from build123d import *

# Parameters (mm, degrees)
SKETCH1_R           = 3.5
BOSS_EXTRUDE1_DEPTH = 17.78
SKETCH2_R           = 12.192
CUT_EXTRUDE1_DEPTH  = 15.24
CUT_EXTRUDE3_REACH  = 49.719
SKETCH4_W           = 2
SKETCH4_H           = 2
CUT_EXTRUDE4_REACH  = 45.308
SKETCH5_R           = 1.5
SKETCH5_W           = 10
SKETCH5_H           = 25.4
CUT_EXTRUDE5_REACH  = 38.451
SKETCH2_2_R         = 12.192
SKETCH6_R           = 12.192
BOSS_EXTRUDE2_DEPTH = 8
CUT_EXTRUDE6_REACH  = 55.634
SKETCH7_W           = 3
SKETCH7_H           = 3


with BuildPart() as part:
    # Sketch1 → Boss-Extrude1 (new, symmetric)
    with BuildSketch(Plane.XY):
        Polygon((26.938, -11.938), (16.938, -11.938), (16.938, 16.938), (-16.938, 16.938), (-16.938, -11.938), (-26.938, -11.938), (-26.938, -16.938), (26.938, -16.938), align=None)
        Circle(SKETCH1_R, mode=Mode.SUBTRACT)
    extrude(amount=BOSS_EXTRUDE1_DEPTH, both=True)

    # Sketch2 → Cut-Extrude1 (cut, symmetric)
    with BuildSketch(Plane.XY):
        Circle(SKETCH2_R)
    extrude(amount=CUT_EXTRUDE1_DEPTH, both=True, mode=Mode.SUBTRACT)

    # Sketch4 → Cut-Extrude3 (cut, up to next)
    with BuildSketch(Plane.XY.offset(17.78), mode=Mode.PRIVATE) as cut_extrude3_sk1:
        with Locations((-10.219, -1)):
            Rectangle(SKETCH4_W, SKETCH4_H)
    cut_extrude3_tool1 = extrude(cut_extrude3_sk1.sketch, amount=-CUT_EXTRUDE3_REACH, mode=Mode.PRIVATE) & part.part
    # Sketch4 → Cut-Extrude3 (cut, up to next)
    with BuildSketch(Plane.XY.offset(17.78), mode=Mode.PRIVATE) as cut_extrude3_sk2:
        with Locations((10.219, -1)):
            Rectangle(SKETCH4_W, SKETCH4_H)
    cut_extrude3_tool2 = extrude(cut_extrude3_sk2.sketch, amount=-CUT_EXTRUDE3_REACH, mode=Mode.PRIVATE) & part.part
    add(cut_extrude3_tool1.solids().sort_by_distance((-10.219, -1, 17.78))[0], mode=Mode.SUBTRACT)
    add(cut_extrude3_tool2.solids().sort_by_distance((10.219, -1, 17.78))[0], mode=Mode.SUBTRACT)

    # Sketch5 → Cut-Extrude4 (cut, up to next)
    with BuildSketch(Plane(origin=(0, -11.938, 0), x_dir=(1, 0, 0), z_dir=(0, 1, 0)), mode=Mode.PRIVATE) as cut_extrude4_sk1:
        with Locations(Location((-21.938, 15.24, 0), (0, 0, 270))):
            Circle(SKETCH5_R)
    cut_extrude4_tool1 = extrude(cut_extrude4_sk1.sketch, amount=-CUT_EXTRUDE4_REACH, mode=Mode.PRIVATE) & part.part
    # Sketch5 → Cut-Extrude4 (cut, up to next)
    with BuildSketch(Plane(origin=(0, -11.938, 0), x_dir=(1, 0, 0), z_dir=(0, 1, 0)), mode=Mode.PRIVATE) as cut_extrude4_sk2:
        with Locations(Location((21.938, 15.24, 0), (0, 0, 90))):
            Circle(SKETCH5_R)
    cut_extrude4_tool2 = extrude(cut_extrude4_sk2.sketch, amount=-CUT_EXTRUDE4_REACH, mode=Mode.PRIVATE) & part.part
    # Sketch5 → Cut-Extrude4 (cut, up to next)
    with BuildSketch(Plane(origin=(0, -11.938, 0), x_dir=(1, 0, 0), z_dir=(0, 1, 0)), mode=Mode.PRIVATE) as cut_extrude4_sk3:
        with Locations(Location((21.938, -15.24, 0), (0, 0, 270))):
            Circle(SKETCH5_R)
    cut_extrude4_tool3 = extrude(cut_extrude4_sk3.sketch, amount=-CUT_EXTRUDE4_REACH, mode=Mode.PRIVATE) & part.part
    # Sketch5 → Cut-Extrude4 (cut, up to next)
    with BuildSketch(Plane(origin=(0, -11.938, 0), x_dir=(1, 0, 0), z_dir=(0, 1, 0)), mode=Mode.PRIVATE) as cut_extrude4_sk4:
        with Locations(Location((-21.938, -15.24, 0), (0, 0, 90))):
            Circle(SKETCH5_R)
    cut_extrude4_tool4 = extrude(cut_extrude4_sk4.sketch, amount=-CUT_EXTRUDE4_REACH, mode=Mode.PRIVATE) & part.part
    # Sketch5 → Cut-Extrude4 (cut, up to next)
    with BuildSketch(Plane(origin=(0, -11.938, 0), x_dir=(1, 0, 0), z_dir=(0, 1, 0)), mode=Mode.PRIVATE) as cut_extrude4_sk5:
        with Locations((-21.938, 0)):
            Rectangle(SKETCH5_W, SKETCH5_H)
    cut_extrude4_tool5 = extrude(cut_extrude4_sk5.sketch, amount=-CUT_EXTRUDE4_REACH, mode=Mode.PRIVATE) & part.part
    # Sketch5 → Cut-Extrude4 (cut, up to next)
    with BuildSketch(Plane(origin=(0, -11.938, 0), x_dir=(1, 0, 0), z_dir=(0, 1, 0)), mode=Mode.PRIVATE) as cut_extrude4_sk6:
        with Locations((21.938, 0)):
            Rectangle(SKETCH5_W, SKETCH5_H)
    cut_extrude4_tool6 = extrude(cut_extrude4_sk6.sketch, amount=-CUT_EXTRUDE4_REACH, mode=Mode.PRIVATE) & part.part
    add(cut_extrude4_tool1.solids().sort_by_distance((-21.938, -11.938, -15.24))[0], mode=Mode.SUBTRACT)
    add(cut_extrude4_tool2.solids().sort_by_distance((21.938, -11.938, -15.24))[0], mode=Mode.SUBTRACT)
    add(cut_extrude4_tool3.solids().sort_by_distance((21.938, -11.938, 15.24))[0], mode=Mode.SUBTRACT)
    add(cut_extrude4_tool4.solids().sort_by_distance((-21.938, -11.938, 15.24))[0], mode=Mode.SUBTRACT)
    add(cut_extrude4_tool5.solids().sort_by_distance((-21.938, -11.938, 0))[0], mode=Mode.SUBTRACT)
    add(cut_extrude4_tool6.solids().sort_by_distance((21.938, -11.938, 0))[0], mode=Mode.SUBTRACT)

    # Sketch2<2> → Cut-Extrude5 (cut, up to next)
    with BuildSketch(Plane.XY, mode=Mode.PRIVATE) as cut_extrude5_sk1:
        Circle(SKETCH2_2_R)
    cut_extrude5_tool1 = extrude(cut_extrude5_sk1.sketch, amount=CUT_EXTRUDE5_REACH, mode=Mode.PRIVATE) & part.part
    add(cut_extrude5_tool1.solids().sort_by_distance((0, 0, 0))[0], mode=Mode.SUBTRACT)

    # Sketch6 → Boss-Extrude2 (add)
    with BuildSketch(Plane.XY.offset(17.78)):
        Polygon((-16.938, -11.938), (-26.938, -11.938), (-26.938, -16.938), (26.938, -16.938), (26.938, -11.938), (16.938, -11.938), (16.938, 16.938), (-16.938, 16.938), align=None)
        Circle(SKETCH6_R, mode=Mode.SUBTRACT)
    extrude(amount=BOSS_EXTRUDE2_DEPTH)

    # Cut-Extrude6: up to this face of the body (flat: up to its plane)
    cut_extrude6_end = Plane(part.part.faces().sort_by_distance((-16.938, 0.946659371, 3.633170238))[0])
    # Sketch7 → Cut-Extrude6 (cut, up to the picked face)
    with BuildSketch(Plane(origin=(16.938, 0, 0), x_dir=(0, 0, -1), z_dir=(1, 0, 0)), mode=Mode.PRIVATE) as cut_extrude6_sk1:
        with Locations((-20.0876, 8.152)):
            Rectangle(SKETCH7_W, SKETCH7_H)
    cut_extrude6_tool1 = split(extrude(cut_extrude6_sk1.sketch, amount=-CUT_EXTRUDE6_REACH, mode=Mode.PRIVATE), bisect_by=cut_extrude6_end, keep=Keep.BOTH, mode=Mode.PRIVATE)
    # Sketch7 → Cut-Extrude6 (cut, up to the picked face)
    with BuildSketch(Plane(origin=(16.938, 0, 0), x_dir=(0, 0, -1), z_dir=(1, 0, 0)), mode=Mode.PRIVATE) as cut_extrude6_sk2:
        with Locations((-20.0876, -8.152)):
            Rectangle(SKETCH7_W, SKETCH7_H)
    cut_extrude6_tool2 = split(extrude(cut_extrude6_sk2.sketch, amount=-CUT_EXTRUDE6_REACH, mode=Mode.PRIVATE), bisect_by=cut_extrude6_end, keep=Keep.BOTH, mode=Mode.PRIVATE)
    add(cut_extrude6_tool1.solids().sort_by(Axis((16.938, 8.152, 20.0876), (-1, 0, 0)))[0], mode=Mode.SUBTRACT)
    add(cut_extrude6_tool2.solids().sort_by(Axis((16.938, -8.152, 20.0876), (-1, 0, 0)))[0], mode=Mode.SUBTRACT)


solid = part.part
CAD build for the part. Positions are in the model's coordinates, mm. A direction names the side the tool comes from. Coordinates: 2 decimals unless noted, no trailing zeros. Write each loop counter-clockwise with the first axis right and the second up, starting at its lowest first coordinate (ties: lowest second). Pieces come first, ordered by that corner, then holes. Notation, with made-up numbers: M 83.5,22.25 L 100.5,22.25 A6 cw 100.5,30.25 Z; hole C 77,-14.75 d9. An arc over 180 degrees is marked long. Answer as a JSON object with one key per item and string values. Group by question number.
1) Saw through at A-A (x = 0). Write the cut outline in (y, z), plus the area to 3 significant figures.
2) Wall check: line 1 (X direction, y = -15.25, z = -15.24); line 2 (Y direction, x = 0, z = 21); line 3 (Z direction, x = 17, y = -12.5). Give the ranges that are in metal, low to high. Write a range as from..to.
3) Mould opens along Z. For faces 3 (the face through (3, -3, -15.24)), 4 (the face through (23.12, -11.938, -14.08)), 5 (the face through (22.85, -14.4, -14.05)) say: +Z half, -Z half, draft (parallel to the pull), parting line (faces both ways), or undercut.
4) Pin check, flat tips, straight feed: pin 1 Ø1.5 at (y, z) = (1.5, 6) entering from +X; pin 2 Ø5.5 at (x, y) = (0, 0) entering from +Z; pin 3 Ø5.5 at (x, z) = (23, -15) entering from +Y; pin 4 Ø5 at (y, z) = (-6.5, 16.5) entering from -X. Stop position of each tip, or through.
5) Saw through at B-B (y = 8). Write the cut outline in (x, z).
6) Tool access for faces 1 (the face through (0, -4, -17.78)), 2 (the face through (-13, -8, 18.588)): list every direction of +Z, -Z, +X, -X, +Y, -Y with a clear straight run to the whole face (end or side of a thin tool).
7) Saw through at D-D (z = 12). Write the cut outline in (x, y).
Values follow:
{
 "1": {"outline": "M -16.94,-17.78 L -3.5,-17.78 L -3.5,-15.24 L -12.19,-15.24 L -12.19,25.78 L -16.94,25.78 Z; M 3.5,-17.78 L 16.94,-17.78 L 16.94,25.78 L 12.19,25.78 L 12.19,-15.24 L 3.5,-15.24 Z", "area": "458 mm2"},
 "2": {"line 1": "x = -26.94..-23.44, -20.44..20.44, 23.44..26.94", "line 2": "y = -16.94..-12.19, 12.19..16.94", "line 3": "z = -17.78..-12.7, 12.7..25.78"},
 "3": {"face 3": "+Z half", "face 4": "draft", "face 5": "undercut"},
 "4": {"pin 1": "stops at x = 16.94", "pin 2": "passes through", "pin 3": "stops at y = -11.94", "pin 4": "stops at x = -16.94"},
 "5": {"outline": "M -16.94,-17.78 L 16.94,-17.78 L 16.94,18.59 L 9.2,18.59 L 9.2,-15.24 L -9.2,-15.24 L -9.2,18.59 L -16.94,18.59 Z; M -16.94,21.59 L -9.2,21.59 L -9.2,25.78 L -16.94,25.78 Z; M 9.2,21.59 L 16.94,21.59 L 16.94,25.78 L 9.2,25.78 Z"},
 "6": {"face 1": "-Z, +X, -X, +Y, -Y", "face 2": "+X, -X"},
 "7": {"outline": "M -16.94,-16.94 L 16.94,-16.94 L 16.94,16.94 L -16.94,16.94 Z; hole C 0,0 d24.38"}
}
